Geometry: see drawing. Coordinates: mm, zero at the bounding-box minimum. Give positions to 0.01 mm unless a question says otherwise; leave off trailing zeros. Write each loop counter-clockwise with the first axis right and the second up, starting at its lowest first coordinate (ties: lowest second). Pieces come first, ordered by that corner, then holes. Notation, with made-up numbers: (18.5, -3) - (36.5, -3) arc R8 ccw to (36.5, 5) - close; hole circle Ø6 at (74, -4). An arc over 180 degrees is marked (long way). Use CSV: the item, a comma, the result in double quotes. Start each with the question number.
(1) First-contact query: pin 1 Ø1 at (y, z) = (47.5, 17.5) entering from -X; pin 2 Ø1.5 at (x, z) = (9.5, 20) entering from +Y (1 decimal); pin 3 Ø8 at (x, z) = (28, 11.5) entering from +Y (1 decimal); pin 4 Ø5 at (x, z) = (7.5, 21.5) entering from +Y (1 decimal). Flat tips, straight axial feed; report the tip coordinate or a pass-through.
(2) Section A-A on z = 20. Output: boundary loops of the cut face in (x, y) (1 decimal).
(3) Section B-B on x = 9. Output: boundary loops of the cut face in (y, z) (1 decimal).
(4) Line query: probe 1 along Y at (x, z) = (2.5, 4.5) (1 decimal); probe 2 along Y at (x, z) = (2, 18) (1 decimal); probe 3 along X at (y, z) = (209, 27) (1 decimal). Output: solid intervals per line, ascending. Write a range as [from, to].
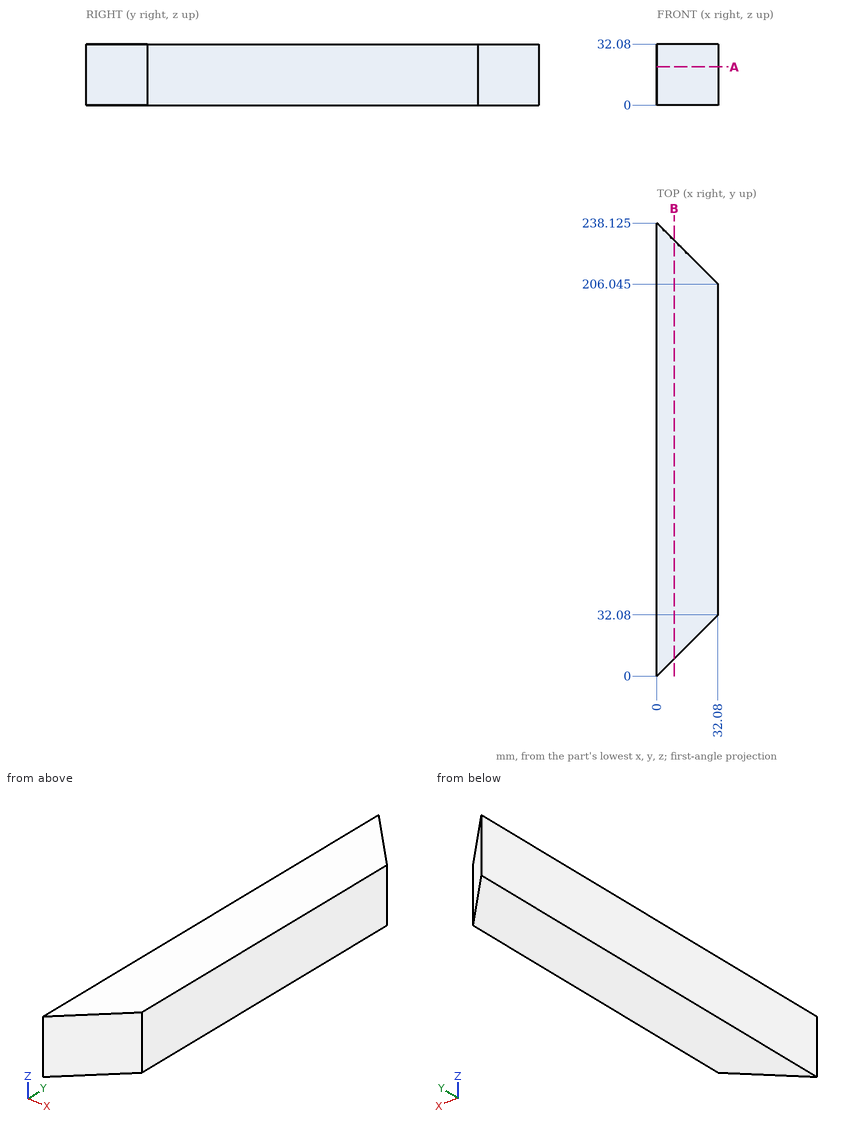
Check values:
1,pin 1,"stops at x = 0"
1,pin 2,"stops at y = 229.4"
1,pin 3,"stops at y = 214.1"
1,pin 4,"stops at y = 233.1"
2,outline,"(0, 0) - (32.1, 32.1) - (32.1, 206) - (0, 238.1) - close"
3,outline,"(9, 0) - (229.1, 0) - (229.1, 32.1) - (9, 32.1) - close"
4,probe 1,"y = [2.5, 235.6]"
4,probe 2,"y = [2, 236.1]"
4,probe 3,"x = [0, 29.1]"
